Design review of the part built by this model. Coordinates are the model's own, in mm. Face numbers are marked on the shaded views. A direction names the side the tool comes from. Give positions to 0.01 mm unless a question says otherwise; leave off trailing zeros. Write each loop counter-clockwise with the first axis right and the second up, starting at its lowest first coordinate (ties: lowest second). Pieces come first, ordered by that corner, then holes.
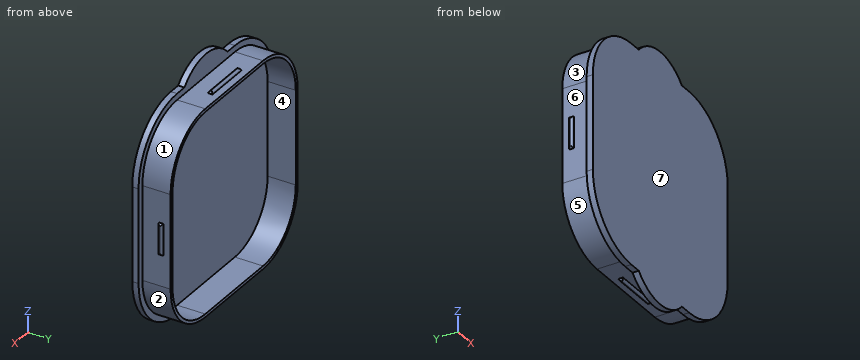
```python
from build123d import *

# Parameters (mm, degrees)
EXTRUDE_1_DEPTH        = 2
FILLET_1_R             = 20
EXTRUDE_2_DEPTH        = 9
CUT_EXTRUDE_2_DEPTH    = 9
SKETCH_4_W             = 10
SKETCH_4_H             = 1.4
EXTRUDE_3_DEPTH        = 0.7
FILLET_2_R             = 0.7
FILLET_2_OF_MIRROR_1_R = 0.7
SKETCH_5_W             = 15
SKETCH_5_H             = 1.4
EXTRUDE_4_DEPTH        = 0.7
FILLET_3_R             = 0.7
FILLET_3_OF_MIRROR_2_R = 0.7


with BuildPart() as part:
    # 草图1 → 凸台-拉伸1 (new body)
    with BuildSketch(Plane(origin=(0, 0, 0), x_dir=(1, 0, 0), z_dir=(0, 1, 0))):
        with BuildLine():
            Line((-35, -35), (-11.180339887, -35))
            ThreePointArc((-11.180339887, -35), (0, -40), (11.180339887, -35))
            Line((11.180339887, -35), (35, -35))
            Line((35, -35), (35, 35))
            Line((35, 35), (11.180339887, 35))
            ThreePointArc((11.180339887, 35), (0, 40), (-11.180339887, 35))
            Line((-11.180339887, 35), (-35, 35))
            Line((-35, 35), (-35, -35))
        make_face()
    extrude(amount=EXTRUDE_1_DEPTH)

    # 圆角1
    fillet_1_edges = [part.edges().sort_by_distance(p)[0] for p in [
        (35, 1, -35),
        (35, 1, 35),
        (-35, 1, 35),
        (-35, 1, -35),
    ]]
    fillet(fillet_1_edges, radius=FILLET_1_R)

    # 草图2 → 凸台-拉伸2 (add)
    with BuildSketch(Plane(origin=(0, 2, 0), x_dir=(1, 0, 0), z_dir=(0, 1, 0))):
        with BuildLine():
            Line((-10.246950766, 33), (10.246950766, 33))
            Line((10.246950766, 33), (15, 33))
            ThreePointArc((15, 33), (27.727922061, 27.727922061), (33, 15))
            Line((33, 15), (33, -15))
            ThreePointArc((33, -15), (27.727922061, -27.727922061), (15, -33))
            Line((15, -33), (10.246950766, -33))
            Line((10.246950766, -33), (-10.246950766, -33))
            Line((-10.246950766, -33), (-15, -33))
            ThreePointArc((-15, -33), (-27.727922061, -27.727922061), (-33, -15))
            Line((-33, -15), (-33, 15))
            ThreePointArc((-33, 15), (-27.727922061, 27.727922061), (-15, 33))
            Line((-15, 33), (-10.246950766, 33))
        make_face()
    extrude(amount=EXTRUDE_2_DEPTH)

    # 草图3 → 切除-拉伸2 (cut)
    with BuildSketch(Plane(origin=(0, 11, 0), x_dir=(1, 0, 0), z_dir=(0, 1, 0))):
        with BuildLine():
            Line((-15, -32), (15, -32))
            ThreePointArc((15, -32), (27.02081528, -27.02081528), (32, -15))
            Line((32, -15), (32, 15))
            ThreePointArc((32, 15), (27.02081528, 27.02081528), (15, 32))
            Line((15, 32), (-15, 32))
            ThreePointArc((-15, 32), (-27.02081528, 27.02081528), (-32, 15))
            Line((-32, 15), (-32, -15))
            ThreePointArc((-32, -15), (-27.02081528, -27.02081528), (-15, -32))
        make_face()
    extrude(amount=-CUT_EXTRUDE_2_DEPTH, mode=Mode.SUBTRACT)

    # 草图4 → 凸台-拉伸3 (add)
    with BuildSketch(Plane.ZY.offset(33)):
        with Locations((0, 8)):
            Rectangle(SKETCH_4_W, SKETCH_4_H)
    extrude_3 = extrude(amount=EXTRUDE_3_DEPTH)

    # 圆角2
    fillet_2_edges = [part.edges().sort_by_distance(p)[0] for p in [
        (-33.7, 8, 5),
        (-33.7, 8, -5),
        (-33.7, 7.3, 0),
        (-33.7, 8.7, 0),
    ]]
    fillet(fillet_2_edges, radius=FILLET_2_R - 0.0001)  # a hair under: the kernel refuses the full size

    # 镜向1: 凸台-拉伸3 across plane
    add(extrude_3.mirror(Plane(origin=(0, 0, 0), x_dir=(0, 0, 1), z_dir=(1, 0, 0))))

    # 圆角2 of 镜向1
    fillet_2_of_mirror_1_edges = [part.edges().sort_by_distance(p)[0] for p in [
        (33.7, 8, 5),
        (33.7, 8, -5),
        (33.7, 7.3, 0),
        (33.7, 8.7, 0),
    ]]
    fillet(fillet_2_of_mirror_1_edges, radius=FILLET_2_OF_MIRROR_1_R - 0.0001)  # a hair under: the kernel refuses the full size

    # 草图5 → 凸台-拉伸4 (add)
    with BuildSketch(Plane.XY.offset(33)):
        with Locations((0, 8)):
            Rectangle(SKETCH_5_W, SKETCH_5_H)
    extrude_4 = extrude(amount=EXTRUDE_4_DEPTH)

    # 圆角3
    fillet_3_edges = [part.edges().sort_by_distance(p)[0] for p in [
        (0, 7.3, 33.7),
        (-7.5, 8, 33.7),
        (0, 8.7, 33.7),
        (7.5, 8, 33.7),
    ]]
    fillet(fillet_3_edges, radius=FILLET_3_R - 0.0001)  # a hair under: the kernel refuses the full size

    # 镜向2: 凸台-拉伸4 across plane
    add(extrude_4.mirror(Plane.XY))

    # 圆角3 of 镜向2
    fillet_3_of_mirror_2_edges = [part.edges().sort_by_distance(p)[0] for p in [
        (0, 7.3, -33.7),
        (-7.5, 8, -33.7),
        (0, 8.7, -33.7),
        (7.5, 8, -33.7),
    ]]
    fillet(fillet_3_of_mirror_2_edges, radius=FILLET_3_OF_MIRROR_2_R - 0.0001)  # a hair under: the kernel refuses the full size


solid = part.part
```
(1) Consider section A-A, the plane z = 13. Give the boundary of the cut face in (x, y).
Resolved:
outline: (-35, 0) - (35, 0) - (35, 2) - (33, 2) - (33, 11) - (32, 11) - (32, 2) - (-32, 2) - (-32, 11) - (-33, 11) - (-33, 2) - (-35, 2) - close
(2) Consider section B-B, the plane y = 5. Give the boundary of the cut face in (x, z), then the cut area to 3 significant figures.
Resolved:
outline: (-33, -15) arc R18 ccw to (-15, -33) - (15, -33) arc R18 ccw to (33, -15) - (33, 15) arc R18 ccw to (15, 33) - (-15, 33) arc R18 ccw to (-33, 15) - close; hole (-32, -15) arc R17 ccw to (-15, -32) - (15, -32) arc R17 ccw to (32, -15) - (32, 15) arc R17 ccw to (15, 32) - (-15, 32) arc R17 ccw to (-32, 15) - close
area: 230 mm2
(3) Tool access review of the marked faces 1, 2, 3 and 4: name each direction out of +Z, -Z, +X, -X, +Y, -Y from which nothing blocks a thin tool from reaching the whole face with its end or side.
Resolved:
face 1: +Z, +X, +Y
face 2: -Z, +X, +Y
face 3: +Z, -X, +Y
face 4: +Y
(4) Mouldability with a two-part tool opening along Y and no side actions: class the marked faces 5, 6 and 7 as pulls with the +Y half, pulls with the -Y half, needs draft (parallel to the pull), parting line crosses it, or undercut.
Resolved:
face 5: needs draft
face 6: undercut
face 7: pulls with the -Y half
(5) To check wall thickness, follow L1, parallel to Z at x = -3.5, y = 2.25; L2, parallel to Z at x = 25, y = 7. State the ranges of each line that lie inside material, in increasing order.
Resolved:
L1: z = -33 to -32, 32 to 33
L2: z = -29.97 to -28.75, 28.75 to 29.97
(6) Consider section C-C, the plane x = -29. Give the boundary of the cut face in (y, z).
Resolved:
outline: (0, -29.28) - (2, -29.28) - (2, -26.31) - (11, -26.31) - (11, -24.64) - (2, -24.64) - (2, 24.64) - (11, 24.64) - (11, 26.31) - (2, 26.31) - (2, 29.28) - (0, 29.28) - close
(7) Clearance check with flat-ended pins moving along their axes: P1, Ø2.5, axis at y = 5.5, z = 4.5, coming from the -X side; P2, Ø5, axis at x = 2.5, y = 4, coming from the +Z side; P3, Ø1.6, axis at x = -14, y = 1, coming from the +Z side. State where each tip first meets the part, or that it passes through.
Resolved:
P1: stops at x = -33
P2: stops at z = 39.97
P3: stops at z = 35
